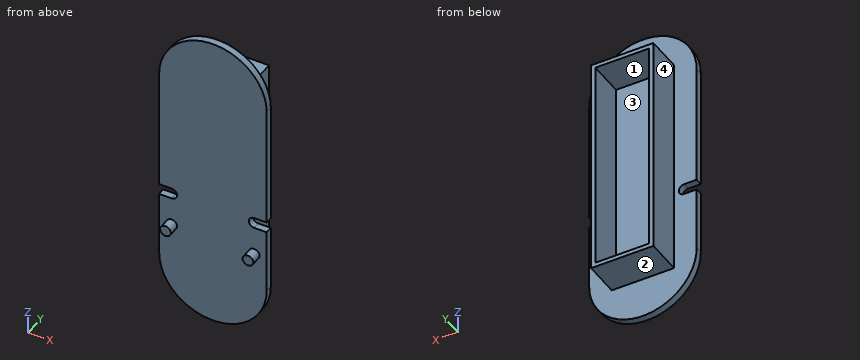
```python
from build123d import *

# Parameters (mm, degrees)
PLATE_EXTRUDE_DEPTH = 2
PEG_SKETCH_R        = 1.5
PEG_EXTRUDE_DEPTH   = 3
SKETCH3_W           = 17.4
SKETCH3_H           = 62.4
SKETCH3_W_2         = 15
SKETCH3_H_2         = 60
BOSS_EXTRUDE3_DEPTH = 10


with BuildPart() as part:
    # Plate Sketch → Plate Extrude (new body)
    with BuildSketch(Plane(origin=(0, 0, 0), x_dir=(1, 0, 0), z_dir=(0, 1, 0))):
        with BuildLine():
            Line((15, 10), (15, -8))
            Line((15, -8), (11.5, -8))
            ThreePointArc((11.5, -8), (10, -9.5), (11.5, -11))
            Line((11.5, -11), (15, -11))
            Line((15, -11), (15, -45))
            ThreePointArc((15, -45), (0, -60), (-15, -45))
            Line((-15, -45), (-15, -11))
            Line((-15, -11), (-11.5, -11))
            ThreePointArc((-11.5, -11), (-10, -9.5), (-11.5, -8))
            Line((-11.5, -8), (-15, -8))
            Line((-15, -8), (-15, 10))
            ThreePointArc((-15, 10), (0, 25), (15, 10))
        make_face()
    extrude(amount=PLATE_EXTRUDE_DEPTH)

    # Peg Sketch → Peg Extrude (add)
    with BuildSketch(Plane.XZ):
        with Locations(Location((11.5, 0, 0), (0, 0, 90))):
            Circle(PEG_SKETCH_R)
        with Locations(Location((-11.5, 0, 0), (0, 0, 90))):
            Circle(PEG_SKETCH_R)
    extrude(amount=PEG_EXTRUDE_DEPTH)

    # Sketch3 → Boss-Extrude3 (add)
    with BuildSketch(Plane(origin=(0, 2, 0), x_dir=(1, 0, 0), z_dir=(0, 1, 0))):
        with Locations((0, -17.5)):
            Rectangle(SKETCH3_W, SKETCH3_H)
        with Locations((0, -17.5)):
            Rectangle(SKETCH3_W_2, SKETCH3_H_2, mode=Mode.SUBTRACT)
    extrude(amount=BOSS_EXTRUDE3_DEPTH)


solid = part.part
```
CAD build for the part. Positions are in the model's coordinates, mm. Face numbers are marked on the shaded views. Round coordinates to 2 decimals unless told otherwise and drop trailing zeros. Order: outer loops, then holes, each group sorted by start corner. A loop starts at its lowest first (then second) coordinate and runs counter-clockwise, first axis right, second up. Notation, with made-up numbers: (-20, 74.25) -> (-9, 74.25) arc R23 cw to (-9, 91.25) -> close; hole circle Ø5 at (-24, 39). An arc over 180 degrees is marked (long way). Write item = value, one per line.
(1) Drill centre lines: L1, parallel to Z at x = 5.5, y = 3.25; L2, parallel to X at y = 4.5, z = -11; L3, parallel to Y at x = 9, z = 43. Where is each one in solid material? Low to high.
Answers follow:
L1 = -13.7 to -12.5, 47.5 to 48.7
L2 = -8.7 to -7.5, 7.5 to 8.7
L3 = 0 to 2
(2) Pull direction X, two halves, no side cores. Call the marked faces 1, 2, 3 and 4: +X half, -X half, draft (parallel to the pull), parting line (faces both ways), or undercut.
Answers follow:
face_1 = undercut
face_2 = draft
face_3 = undercut
face_4 = -X half
(3) Cut at C-C (x = 0). Write the cut outline in (y, z), plus the area to 3 significant figures.
Answers follow:
outline = (0, -25) -> (2, -25) -> (2, -13.7) -> (12, -13.7) -> (12, -12.5) -> (2, -12.5) -> (2, 47.5) -> (12, 47.5) -> (12, 48.7) -> (2, 48.7) -> (2, 60) -> (0, 60) -> close
area = 194 mm²
(4) Cut at B-B (z = 9.5). Write the cut outline in (x, y), plus the area to 3 significant figures.
Answers follow:
outline = (-10, 0) -> (10, 0) -> (10, 2) -> (8.7, 2) -> (8.7, 12) -> (7.5, 12) -> (7.5, 2) -> (-7.5, 2) -> (-7.5, 12) -> (-8.7, 12) -> (-8.7, 2) -> (-10, 2) -> close
area = 64.0 mm²
(5) Cut at A-A (y = 5.5). Write the cut outline in (x, z).
Answers follow:
outline = (-8.7, -13.7) -> (8.7, -13.7) -> (8.7, 48.7) -> (-8.7, 48.7) -> close; hole (-7.5, -12.5) -> (7.5, -12.5) -> (7.5, 47.5) -> (-7.5, 47.5) -> close
(6) Cut at D-D (y = -2). Write the cut outline in (x, z).
Answers follow:
outline = circle Ø3 at (-11.5, 0); circle Ø3 at (11.5, 0)
(7) Flat gauge pins, fed straight in: P1, Ø2, axis at x = 12.5, y = 1.5, coming from the -Z side; P2, Ø2, axis at x = -12.5, y = 1.5, coming from the +Z side; P3, Ø10, axis at x = -9.5, z = 26.5, coming from the +Y side; P4, Ø5, axis at x = 6.5, y = -0.5, coming from the +Z side. Where does each tip first touch, or does it go through?
Answers follow:
P1 = -19.63
P2 = 54.63
P3 = 12
P4 = 59.44
